The model under review builds one solid part; all positions refer to its coordinate system, in mm. Coordinates: 2 decimals unless noted, no trailing zeros. Loops run counter-clockwise (first coordinate to the right, second up) from the corner with the lowest first, then second, coordinate; pieces in that order, holes last. Notation, with made-up numbers: M 77.5,-17.75 L 118.5,-17.75 A24 ccw 118.5,3.25 Z; hole C -1,47.25 d3. An arc over 180 degrees is marked long. Return JSON: item names as keys, results as strings.
```python
from build123d import *

# Parameters (mm, degrees)
F0_R     = 4
F1_DEPTH = 1


with BuildPart() as f1:
    # F0 (on Right) → F1 (new body)
    with BuildSketch(Plane.YZ):
        with BuildLine():
            ThreePointArc((6.502189, -7.407407), (5.079872, 0), (6.502189, 7.407407))
            ThreePointArc((6.502189, 7.407407), (0, 17), (-6.502189, 7.407407))
            ThreePointArc((-6.502189, 7.407407), (-5.079872, 0), (-6.502189, -7.407407))
            ThreePointArc((-6.502189, -7.407407), (0, -17), (6.502189, -7.407407))
        make_face()
        with Locations((0, -10)):
            Circle(F0_R, mode=Mode.SUBTRACT)
        with Locations((0, 10)):
            Circle(F0_R, mode=Mode.SUBTRACT)
    extrude(amount=F1_DEPTH)


solid = f1.part
```
1. The part is to be moulded in two halves that separate along Z. For faces 1 (the face through (1, 0, 0)), 2 (the face through (0.493, -0.521, 13.966)), say which applies: released by +Z, released by -Z, zero draft, split by the parting line, or undercut.
Check values:
{"face 1": "zero draft", "face 2": "undercut"}
2. Add section A-A on y = 0. Give the boundary of the cut face in (x, z).
Check values:
{"outline": "M 0,-17 L 1,-17 L 1,-14 L 0,-14 Z; M 0,-6 L 1,-6 L 1,6 L 0,6 Z; M 0,14 L 1,14 L 1,17 L 0,17 Z"}
3. Add section C-C on y = -6. Give the boundary of the cut face in (x, z).
Check values:
{"outline": "M 0,-13.61 L 1,-13.61 L 1,-6 L 0,-6 Z; M 0,6 L 1,6 L 1,13.61 L 0,13.61 Z"}
4. To check wall thickness, follow line 1 (Z direction, x = 0.4, y = 0); line 2 (Z direction, x = 0.7, y = 2.75); line 3 (Y direction, x = 0.9, z = 9.5). State the ranges of each line that lie inside material, in increasing order.
Check values:
{"line 1": "-17 to -14, -6 to 6, 14 to 17", "line 2": "-16.44 to -12.9, -7.1 to 7.1, 12.9 to 16.44", "line 3": "-6.98 to -3.97, 3.97 to 6.98"}
5. Add section B-B on z = 10. Give the boundary of the cut face in (x, y), plus the area to 3 significant figures.
Check values:
{"outline": "M 0,-7 L 1,-7 L 1,-4 L 0,-4 Z; M 0,4 L 1,4 L 1,7 L 0,7 Z", "area": "6.00 mm²"}
6. Add section D-D on x = 0.7. Give the boundary of the cut face in (y, z), plus the area to 3 significant figures.
Check values:
{"outline": "M -6.5,-7.41 A7 ccw long 6.5,-7.41 A20 cw 6.5,7.41 A7 ccw long -6.5,7.41 A20 cw Z; hole C 0,-10 d8; hole C 0,10 d8", "area": "289 mm²"}
